Input: part model. Units: mm. Frame: model coordinates. A direction names the side the tool comes from. Round coordinates to 2 decimals unless told otherwise and drop trailing zeros. Order: outer loops, then holes, each group sorted by start corner. A loop starts at its lowest first (then second) coordinate and runs counter-clockwise, first axis right, second up. Notation, with made-up numbers: (85, 47.25) -> (123, 47.25) arc R21 ccw to (123, 65.25) -> close; hole circle Ø8 at (-34.75, -7). An arc over 180 degrees is marked (long way). Use a Markdown table: item, result.
from build123d import *

# Parameters (mm, degrees)
F0_W           = 38.5
F0_H           = 39.4
F0_R           = 1.6
F1_DEPTH       = 3
F0_R_2         = 0.8
F2_DEPTH       = 11.4
F3_DEPTH       = 16
F0_R_3         = 1.25
F4_DEPTH       = 38
F5_W           = 1.25
F5_H           = 5
F6_DEPTH       = 28
F10_DEPTH      = 19.25
F10_DEPTH_BACK = 19.25


with BuildPart() as f1:
    # F0 (on Top) → F1 (new body)
    with BuildSketch(Plane.XY):
        Rectangle(F0_W, F0_H)
        with Locations((-14.25, -14.25)):
            Circle(F0_R, mode=Mode.SUBTRACT)
        with Locations((14.25, -14.25)):
            Circle(F0_R, mode=Mode.SUBTRACT)
        with Locations((-14.25, 14.25)):
            Circle(F0_R, mode=Mode.SUBTRACT)
        with Locations((14.25, 14.25)):
            Circle(F0_R, mode=Mode.SUBTRACT)
    extrude(amount=F1_DEPTH)

    # F0 (on Top) → F2 (join)
    with BuildSketch(Plane.XY):
        with Locations((-14.25, 14.25)):
            Circle(F0_R)
        with Locations((-14.25, 14.25)):
            Circle(F0_R_2, mode=Mode.SUBTRACT)
        with Locations((-14.25, -14.25)):
            Circle(F0_R)
        with Locations((-14.25, -14.25)):
            Circle(F0_R_2, mode=Mode.SUBTRACT)
        with Locations((14.25, -14.25)):
            Circle(F0_R)
        with Locations((14.25, -14.25)):
            Circle(F0_R_2, mode=Mode.SUBTRACT)
        with Locations((14.25, 14.25)):
            Circle(F0_R)
        with Locations((14.25, 14.25)):
            Circle(F0_R_2, mode=Mode.SUBTRACT)
    extrude(amount=F2_DEPTH)

    # F0 (on Top) → F3 (join)
    with BuildSketch(Plane.XY):
        with Locations((-14.25, 14.25)):
            Circle(F0_R_2)
        with Locations((-14.25, -14.25)):
            Circle(F0_R_2)
        with Locations((14.25, -14.25)):
            Circle(F0_R_2)
        with Locations((14.25, 14.25)):
            Circle(F0_R_2)
    extrude(amount=F3_DEPTH)

    # F0 (on Top) → F4 (join)
    with BuildSketch(Plane.XY):
        Polygon((20.5, 21), (-20.5, 21), (-20.5, 6), (-20.5, -6), (-20.5, -21), (20.5, -21), (20.5, -6), (20.5, 6), align=None)
        Rectangle(F0_W, F0_H, mode=Mode.SUBTRACT)
        with BuildLine():
            Line((-20.5, -21), (-20.5, -6))
            ThreePointArc((-20.5, -6), (-28, -13.5), (-20.5, -21))
        make_face()
        with Locations((-24.25, -13.5)):
            Circle(F0_R_3, mode=Mode.SUBTRACT)
        with BuildLine():
            ThreePointArc((20.5, -21), (28, -13.5), (20.5, -6))
            Line((20.5, -6), (20.5, -21))
        make_face()
        with Locations((24.25, -13.5)):
            Circle(F0_R_3, mode=Mode.SUBTRACT)
        with BuildLine():
            ThreePointArc((20.5, 6), (28, 13.5), (20.5, 21))
            Line((20.5, 21), (20.5, 6))
        make_face()
        with Locations((24.25, 13.5)):
            Circle(F0_R_3, mode=Mode.SUBTRACT)
        with BuildLine():
            Line((-20.5, 6), (-20.5, 21))
            ThreePointArc((-20.5, 21), (-28, 13.5), (-20.5, 6))
        make_face()
        with Locations((-24.25, 13.5)):
            Circle(F0_R_3, mode=Mode.SUBTRACT)
    extrude(amount=F4_DEPTH)

    # F5 (on face) → F6 (cut)
    with BuildSketch(Plane.XY.offset(38)):
        with Locations((-19.875, 0)):
            Rectangle(F5_W, F5_H)
    extrude(amount=-F6_DEPTH, mode=Mode.SUBTRACT)

    # F9 (on Right) → F10 (join, two sides)
    with BuildSketch(Plane.YZ) as f10_sk:
        with BuildLine():
            Line((19.7, 13), (19.7, 15))
            ThreePointArc((19.7, 15), (19.110149, 14), (19.7, 13))
        make_face()
        with BuildLine():
            ThreePointArc((-19.7, 13), (-19.110149, 14), (-19.7, 15))
            Line((-19.7, 15), (-19.7, 13))
        make_face()
    extrude(amount=F10_DEPTH)
    extrude(f10_sk.sketch, amount=-F10_DEPTH_BACK)


solid = f1.part
1) Contact query for flat-ended pins moving along their axis: P1, Ø1.5, axis at y = 3.5, z = 30, coming from the -X side; P2, Ø3, axis at x = -17, y = 11.5, coming from the +Z side; P3, Ø2.5, axis at x = 13.5, y = 14, coming from the +Z side. Output: stop coordinate, or through.
Answer key:
| item | result |
|---|---|
| P1 | stops at x = -20.5 |
| P2 | stops at z = 3 |
| P3 | stops at z = 16 |
2) Cut plane B-B on y = -18. Return loops of the section in (x, z).
Answer key:
| item | result |
|---|---|
| outline | (-26.5, 0) -> (26.5, 0) -> (26.5, 38) -> (19.25, 38) -> (19.25, 3) -> (-19.25, 3) -> (-19.25, 38) -> (-26.5, 38) -> close |
3) Set-up query: faces 1 (the face through (-15.85, 14.32, 7.14)), 2 (the face through (-20.5, -3, 19)), 3 (the face through (0, 19.7, 8)), 4 (the face through (-20, -2.5, 24)), 5 (the face through (-23.578, -12.446, 18.734)). Return all of +Z, -Z, +X, -X, +Y, -Y with unobstructed straight access to the full face (end or side cutting, diameter ignored); none if empty.
Answer key:
| item | result |
|---|---|
| face 1 | +Z |
| face 2 | +Z, -Z, -X |
| face 3 | none |
| face 4 | +Z, -X |
| face 5 | +Z, -Z |
4) Cut plane D-D on x = 14.25. Return loops of the section in (y, z).
Answer key:
| item | result |
|---|---|
| outline | (-21, 0) -> (21, 0) -> (21, 38) -> (19.7, 38) -> (19.7, 15) arc R1.14 ccw to (19.7, 13) -> (19.7, 3) -> (15.85, 3) -> (15.85, 11.4) -> (15.05, 11.4) -> (15.05, 16) -> (13.45, 16) -> (13.45, 11.4) -> (12.65, 11.4) -> (12.65, 3) -> (-12.65, 3) -> (-12.65, 11.4) -> (-13.45, 11.4) -> (-13.45, 16) -> (-15.05, 16) -> (-15.05, 11.4) -> (-15.85, 11.4) -> (-15.85, 3) -> (-19.7, 3) -> (-19.7, 13) arc R1.14 ccw to (-19.7, 15) -> (-19.7, 38) -> (-21, 38) -> close |
5) Cut plane A-A on z = 8. State how many separate pieces and enclosed holes the cut face has, and give its area (3 significant figures).
Answer key:
| item | result |
|---|---|
| separate pieces | 5 |
| enclosed holes | 5 |
| area | 571 mm^2 |
6) Draft query along Y for faces 6 (the face through (0, -21, 19)), 7 (the face through (24.922, 14.554, 18.734)), 8 (the face through (20.5, 0, 19)), 9 (the face through (0, -20, 38)). Return one class per face: released by +Y, released by -Y, zero draft, split by the parting line, or undercut.
Answer key:
| item | result |
|---|---|
| face 6 | released by -Y |
| face 7 | undercut |
| face 8 | undercut |
| face 9 | zero draft |
7) Cut plane C-C on z = 22.5. Return loops of the section in (x, y), and give its area (3 significant figures).
Answer key:
| item | result |
|---|---|
| outline | (-20.5, -21) -> (20.5, -21) arc R7.5 ccw to (20.5, -6) -> (20.5, 6) arc R7.5 ccw to (20.5, 21) -> (-20.5, 21) arc R7.5 ccw to (-20.5, 6) -> (-20.5, 2.5) -> (-19.25, 2.5) -> (-19.25, 19.7) -> (19.25, 19.7) -> (19.25, -19.7) -> (-19.25, -19.7) -> (-19.25, -2.5) -> (-20.5, -2.5) -> (-20.5, -6) arc R7.5 ccw to start; hole circle Ø2.5 at (-24.25, -13.5); hole circle Ø2.5 at (-24.25, 13.5); hole circle Ø2.5 at (24.25, -13.5); hole circle Ø2.5 at (24.25, 13.5) |
| area | 533 mm^2 |
8) Ray query, probe 1 along X at (y, z) = (-13, 20); probe 2 along Y at (x, z) = (24.25, 10); probe 3 along Y at (x, z) = (24, 13). Return the intervals inside material, ascending.
Answer key:
| item | result |
|---|---|
| probe 1 | x = -27.98 to -25.4, -23.1 to -19.25, 19.25 to 23.1, 25.4 to 27.98 |
| probe 2 | y = -20 to -14.75, -12.25 to -7, 7 to 12.25, 14.75 to 20 |
| probe 3 | y = -20.13 to -14.72, -12.28 to -6.87, 6.87 to 12.28, 14.72 to 20.13 |
